```python
from build123d import *

# Parameters (mm, degrees)
REDONDEO1_R = 1


with BuildPart() as part:
    # Croquis1 → Revolución1 (revolve)
    with BuildSketch(Plane.XY, mode=Mode.PRIVATE) as revoluci_n1_sk:
        Polygon((-8.030896413, 0.557253855), (-8.030896413, 1.445392264), (-8.708681637, 2.358698791), (-8.708681637, 4.539307424), (-11.015589151, 4.539307424), (-11.937259367, 3.895637734), (-11.937259367, 1.322020013), (-8.708681637, 1.322020013), align=None)
    revolve(revoluci_n1_sk.sketch.rotate(Axis((0, 26.098695966, 0), (0, -1, 0)), 270), axis=Axis((0, 26.098695966, 0), (0, -1, 0)))

    # Redondeo1
    redondeo1_edges = [part.edges().sort_by_distance(p)[0] for p in [
        (0, 1.322020013, -8.708681637),
    ]]
    fillet(redondeo1_edges, radius=REDONDEO1_R)


solid = part.part
```
For this review, take the finished solid that the model builds, in its own axes (mm). A direction names the side the tool comes from. Coordinates: 2 decimals unless noted, no trailing zeros. Loops run counter-clockwise (first coordinate to the right, second up) from the corner with the lowest first, then second, coordinate; pieces in that order, holes last.
1. For faces 1 (the cylindrical face through (7.726, 3.464, 4.019)), 2 (the flat face through (9, 1.322, -3)), list the 3-axis set-ups (+Z, -Z, +X, -X, +Y, -Y) from which the entire face can be reached by the end or side of a thin tool; tool diameter is ignored.
2. Add section A-A, the plane x = 0. Give the boundary of the cut face in (y, z).
3. Mouldability with a two-part tool opening along X and no side actions: class faces 3 (the cylindrical face through (4.57, 2.59, 11.03)), 4 (the flat face through (-9, 4.539, -1)), 5 (the cylindrical face through (4.89, 1.01, -6.37)) as +X half, -X half, draft (parallel to the pull), parting line (faces both ways), or undercut.
4. For line 1 (X direction, y = 3.8, z = 0); line 2 (X direction, y = 3.2, z = 6); line 3 (Y direction, x = 5, z = -8.25), list the stretches that pass through material, from the lowest coordinate up.
5. Add section B-B, the plane z = 0. Give the boundary of the cut face in (x, y), then the cut area to 3 significant figures.
6. Add section C-C, the plane y = 3.3. Give the boundary of the cut face in (x, z).
Result:
1. face 1: +Y
1. face 2: -Y
2. outline: (0.56, -8.03) - (0.99, -8.41) arc R1 cw to (1.32, -9.16) - (1.32, -11.94) - (3.9, -11.94) - (4.54, -11.02) - (4.54, -8.71) - (2.36, -8.71) - (1.45, -8.03) - close; (0.56, 8.03) - (1.45, 8.03) - (2.36, 8.71) - (4.54, 8.71) - (4.54, 11.02) - (3.9, 11.94) - (1.32, 11.94) - (1.32, 9.16) arc R1 cw to (0.99, 8.41) - close
3. face 3: parting line
3. face 4: draft
3. face 5: undercut
4. line 1: x = -11.94 to -8.71, 8.71 to 11.94
4. line 2: x = -10.32 to -6.31, 6.31 to 10.32
4. line 3: y = 1.32 to 4.54
5. outline: (-11.94, 1.32) - (-9.16, 1.32) arc R1 cw to (-8.41, 0.99) - (-8.03, 0.56) - (-8.03, 1.45) - (-8.71, 2.36) - (-8.71, 4.54) - (-11.02, 4.54) - (-11.94, 3.9) - close; (8.03, 0.56) - (8.41, 0.99) arc R1 cw to (9.16, 1.32) - (11.94, 1.32) - (11.94, 3.9) - (11.02, 4.54) - (8.71, 4.54) - (8.71, 2.36) - (8.03, 1.45) - close
5. area: 21.5 mm2
6. outline: circle Ø23.87 at (0, 0); hole circle Ø17.42 at (0, 0)
